Check sheet for the modelled part. Datum: model origin and axes. Units: mm. Coordinates: 2 decimals unless noted, no trailing zeros. Write each loop counter-clockwise with the first axis right and the second up, starting at its lowest first coordinate (ties: lowest second). Pieces come first, ordered by that corner, then holes. Notation, with made-up numbers: M 74,7.5 L 120,7.5 A26 cw 120,39.5 Z; hole C -24.5,-25 d3. An arc over 180 degrees is marked long. Answer as CSV lines item,"result". Start each with the question number.
1) Go/stop test with flat-tipped pins: pin 1 Ø1 at (y, z) = (-2, 28.5) entering from -X; pin 2 Ø1.9 at (x, y) = (0, 0) entering from +Z (3 decimals); pin 3 Ø2.5 at (x, y) = (0.5, 2) entering from -Z (3 decimals). Record where each tip stops, or that it passes through.
2) Section check C-C (y = 2.5). Record the cut outline in (x, z) (3 decimals), and give its area (3 significant figures).
3) Section check D-D (x = 2.5). Record the cut outline in (y, z) (1 decimal).
4) Section check B-B (x = -2.25). Record the cut outline in (y, z) (1 decimal).
5) Material ranges on L1, parallel to X at y = 0, z = 18.5 (1 decimal); L2, parallel to Z at x = 1.75, y = -1.5 (3 decimals), recorded low to high. Write a range as [from, to].
from build123d import *

# Parameters (mm, degrees)
BOSS_EXTRUDE1_DEPTH      = 0.3175
BOSS_EXTRUDE1_DEPTH_BACK = 0.3175


with BuildPart() as part:
    # Sketch1 → Revolve6 (revolve)
    with BuildSketch(Plane(origin=(0, 0, 0), x_dir=(1, 0, 0), z_dir=(0, 1, 0))):
        Polygon((-3.175, -47.169090574), (-1.5875, -47.169090574), (-1.5875, -28.575), (-1.5875, -3.175), (-3.175, -3.175), align=None)
    revolve(axis=Axis((0, 0, 0), (0, 0, 1)))

    # Sketch1_10 → Boss-Extrude1 (add, two sides)
    with BuildSketch(Plane(origin=(0, 0, 0), x_dir=(1, 0, 0), z_dir=(0, 1, 0))) as boss_extrude1_sk:
        with BuildLine():
            ThreePointArc((-1.5875, -2.749630657), (-0.821750468, -3.066814498), (0, -3.175))
            Line((0, -3.175), (0, -1.27))
            ThreePointArc((0, -1.27), (-1.27, 0), (0, 1.27))
            Line((0, 1.27), (0, 2.749630657))
            Line((0, 2.749630657), (-1.5875, 2.749630657))
            Line((-1.5875, 2.749630657), (-1.5875, -2.749630657))
        make_face()
        with BuildLine():
            Line((0, -1.27), (0, -3.175))
            ThreePointArc((0, -3.175), (0.821750468, -3.066814498), (1.5875, -2.749630657))
            Line((1.5875, -2.749630657), (1.5875, 2.749630657))
            Line((1.5875, 2.749630657), (0, 2.749630657))
            Line((0, 2.749630657), (0, 1.27))
            ThreePointArc((0, 1.27), (0.898025612, 0.898025612), (1.27, 0))
            ThreePointArc((1.27, 0), (0.898025612, -0.898025612), (0, -1.27))
        make_face()
        with BuildLine():
            ThreePointArc((0, 3.175), (-0.821750468, 3.066814498), (-1.5875, 2.749630657))
            Line((-1.5875, 2.749630657), (0, 2.749630657))
            Line((0, 2.749630657), (0, 3.175))
        make_face()
        with BuildLine():
            Line((0, 2.749630657), (1.5875, 2.749630657))
            ThreePointArc((1.5875, 2.749630657), (0.821750468, 3.066814498), (0, 3.175))
            Line((0, 3.175), (0, 2.749630657))
        make_face()
        with BuildLine():
            ThreePointArc((0, 3.175), (-0.821750468, 3.066814498), (-1.5875, 2.749630657))
            Line((-1.5875, 2.749630657), (0, 2.749630657))
            Line((0, 2.749630657), (0, 3.175))
        make_face()
        with BuildLine():
            Line((0, 2.749630657), (1.5875, 2.749630657))
            ThreePointArc((1.5875, 2.749630657), (0.821750468, 3.066814498), (0, 3.175))
            Line((0, 3.175), (0, 2.749630657))
        make_face()
        with BuildLine():
            ThreePointArc((-3.175, 0), (-2.749630657, -1.5875), (-1.5875, -2.749630657))
            Line((-1.5875, -2.749630657), (-1.5875, 2.749630657))
            ThreePointArc((-1.5875, 2.749630657), (-2.749630657, 1.5875), (-3.175, 0))
        make_face()
        with BuildLine():
            Line((1.5875, 2.749630657), (1.5875, -2.749630657))
            ThreePointArc((1.5875, -2.749630657), (2.749630657, -1.5875), (3.175, 0))
            ThreePointArc((3.175, 0), (2.749630657, 1.5875), (1.5875, 2.749630657))
        make_face()
        with BuildLine():
            Line((1.5875, -3.175), (3.175, -3.175))
            Line((3.175, -3.175), (3.175, 0))
            ThreePointArc((3.175, 0), (2.749630657, -1.5875), (1.5875, -2.749630657))
            Line((1.5875, -2.749630657), (1.5875, -3.175))
        make_face()
        with BuildLine():
            ThreePointArc((1.5875, -2.749630657), (0.821750468, -3.066814498), (0, -3.175))
            Line((0, -3.175), (1.5875, -3.175))
            Line((1.5875, -3.175), (1.5875, -2.749630657))
        make_face()
        with BuildLine():
            Line((-1.5875, -2.749630657), (-1.5875, -3.175))
            Line((-1.5875, -3.175), (0, -3.175))
            ThreePointArc((0, -3.175), (-0.821750468, -3.066814498), (-1.5875, -2.749630657))
        make_face()
        with BuildLine():
            Line((-3.175, -3.175), (-1.5875, -3.175))
            Line((-1.5875, -3.175), (-1.5875, -2.749630657))
            ThreePointArc((-1.5875, -2.749630657), (-2.749630657, -1.5875), (-3.175, 0))
            Line((-3.175, 0), (-3.175, -3.175))
        make_face()
    extrude(amount=BOSS_EXTRUDE1_DEPTH)
    extrude(boss_extrude1_sk.sketch, amount=-BOSS_EXTRUDE1_DEPTH_BACK)


solid = part.part
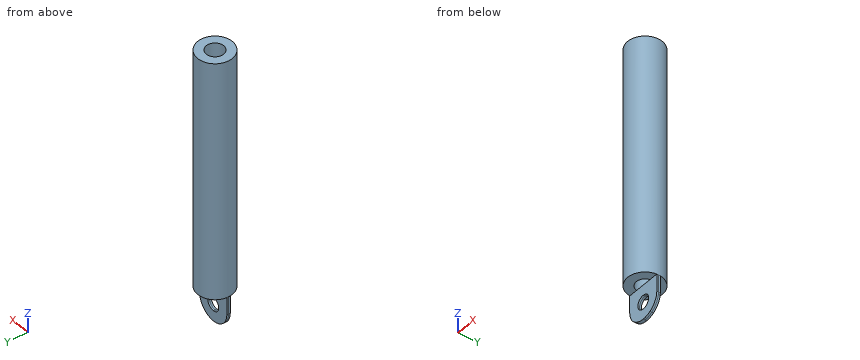
Results found:
1,pin 1,"stops at x = -2.8"
1,pin 2,"stops at z = 3.175"
1,pin 3,"stops at z = 3.175"
2,outline,"M -1.957,3.175 L 1.957,3.175 L 1.957,47.169 L -1.957,47.169 Z"
2,area,"172 mm2"
3,outline,"M -2,3.2 L -0.3,3.2 L -0.3,-2 L 0.3,-2 L 0.3,3.2 L 2,3.2 L 2,47.2 L -2,47.2 Z"
4,outline,"M -2.2,3.2 L -0.3,3.2 L -0.3,-2.2 L 0.3,-2.2 L 0.3,3.2 L 2.2,3.2 L 2.2,47.2 L -2.2,47.2 Z"
5,L1,"x = [-3.2, -1.6], [1.6, 3.2]"
5,L2,"z = [3.175, 47.169]"
